The listing builds one solid part. Answer for the finished solid, in the listing's coordinates (mm). A direction names the side the tool comes from. Give positions to 0.01 mm unless a question says otherwise; leave off trailing zeros. Order: outer loops, then holes, each group sorted by start corner. A loop starts at its lowest first (then second) coordinate and runs counter-clockwise, first axis right, second up. Notation, with made-up numbers: (0.5, 21) - (13.5, 21) arc R26 cw to (13.5, 57) - close; hole circle Ø11 at (-36, 22). An arc over 180 degrees is marked (long way). Answer in a Markdown table with one row per item. Add a question column.
```python
from build123d import *

# Parameters (mm, degrees)
SKETCH1_W           = 68
SKETCH1_H           = 39.37
SKETCH1_R           = 4.25
BOSS_EXTRUDE1_DEPTH = 5
SKETCH2_W           = 68
SKETCH2_H           = 4.7625
BOSS_EXTRUDE2_DEPTH = 68
SKETCH4_R           = 3.15
CUT_EXTRUDE2_DEPTH  = 88.650893072
SKETCH14_R          = 23.5
CUT_EXTRUDE3_DEPTH  = 90.638144224


with BuildPart() as part:
    # Sketch1 → Boss-Extrude1 (new body)
    with BuildSketch(Plane(origin=(0, 0, 0), x_dir=(0, 0, -1), z_dir=(0, 1, 0))):
        Rectangle(SKETCH1_W, SKETCH1_H)
        with Locations(Location((-25, -2.735, 0), (0, 0, 180))):
            Circle(SKETCH1_R, mode=Mode.SUBTRACT)
        with Locations(Location((25, -2.735, 0), (0, 0, 180))):
            Circle(SKETCH1_R, mode=Mode.SUBTRACT)
    extrude(amount=BOSS_EXTRUDE1_DEPTH)

    # Sketch2 → Boss-Extrude2 (add)
    with BuildSketch(Plane(origin=(0, 5, 0), x_dir=(0, 0, -1), z_dir=(0, 1, 0))):
        with Locations((0, 17.30375)):
            Rectangle(SKETCH2_W, SKETCH2_H)
    extrude(amount=BOSS_EXTRUDE2_DEPTH)

    # Sketch4 → Cut-Extrude2 (cut, through all)
    with BuildSketch(Plane(origin=(-14.9225, 0, 0), x_dir=(0, 0, -1), z_dir=(1, 0, 0))):
        with Locations(Location((-27.577164466, 61.577164466, 0), (0, 0, 90))):
            Circle(SKETCH4_R)
        with Locations(Location((27.577164466, 61.577164466, 0), (0, 0, 90))):
            Circle(SKETCH4_R)
    extrude(amount=-CUT_EXTRUDE2_DEPTH, mode=Mode.SUBTRACT)

    # Sketch14 → Cut-Extrude3 (cut, through all)
    with BuildSketch(Plane.ZY.offset(19.685)):
        with Locations((0, 34)):
            Circle(SKETCH14_R)
    extrude(amount=-CUT_EXTRUDE3_DEPTH, mode=Mode.SUBTRACT)


solid = part.part
```
(1) Each of these flat-tipped pins is pushed along its axis until it touches: P1, Ø8, axis at x = 11, z = 26.5, coming from the +Y side; P2, Ø5, axis at y = 59, z = -27, coming from the +X side; P3, Ø5.5, axis at y = 61.58, z = 27.58, coming from the -X side. Where does it stop, or does it pass through?
(2) Find section C-C, the plane y = 34. Write down the section's boundary in (x, z) (1 decimal), plus the area to 3 significant figures.
(3) The mould has two halves that part along Y. Classify faces 1 (the face through (-17.34, 57.3, -3.06)), 2 (the face through (-1.414, 2.465, 24.079)), 3 (the face through (2, 5, 0)): +Y half, -Y half, draft (parallel to the pull), parting line (faces both ways), or undercut.
(4) Find section A-A, the plane y = 61.5. Write down the section's boundary in (x, z) (1 decimal).
(5) Find section D-D, the plane z = -19.5. Write down the section's boundary in (x, y) (1 decimal).
(6) Straight lines are drawn through the part: line 1 (Y direction, x = -15, z = 0); line 2 (Y direction, x = -0.5, z = -11.5); line 3 (X direction, y = 8, z = 23) (1 decimal). For each, find the intervals that lie inside material, in ascending order.
(7) For faces 4 (the face through (19.685, 2, 0)), 5 (the face through (-14.923, 54, 16)), determine the directions among +Z, -Z, +X, -X, +Y, -Y from which every point of the face is accessible in a straight line to the end or side of a thin tool.
(8) Find section B-B, the plane z = 0. Write down the section's boundary in (x, y) (1 decimal).
Answer key:
| question | item | result |
|---|---|---|
| 1 | P1 | y = 5 |
| 1 | P2 | x = -14.92 |
| 1 | P3 | through |
| 2 | outline | (-19.7, -34) - (-14.9, -34) - (-14.9, -23.5) - (-19.7, -23.5) - close; (-19.7, 23.5) - (-14.9, 23.5) - (-14.9, 34) - (-19.7, 34) - close |
| 2 | area | 100 mm² |
| 3 | face 1 | undercut |
| 3 | face 2 | draft |
| 3 | face 3 | +Y half |
| 4 | outline | (-19.7, -34) - (-14.9, -34) - (-14.9, -30.7) - (-19.7, -30.7) - close; (-19.7, -24.4) - (-14.9, -24.4) - (-14.9, 24.4) - (-19.7, 24.4) - close; (-19.7, 30.7) - (-14.9, 30.7) - (-14.9, 34) - (-19.7, 34) - close |
| 5 | outline | (-19.7, 0) - (19.7, 0) - (19.7, 5) - (-14.9, 5) - (-14.9, 20.9) - (-19.7, 20.9) - close; (-19.7, 47.1) - (-14.9, 47.1) - (-14.9, 73) - (-19.7, 73) - close |
| 6 | line 1 | 0 to 10.5, 57.5 to 73 |
| 6 | line 2 | 0 to 5 |
| 6 | line 3 | -19.7 to -14.9 |
| 7 | face 4 | +Z, -Z, +X, +Y, -Y |
| 7 | face 5 | +Z, -Z, +X, +Y |
| 8 | outline | (-19.7, 0) - (19.7, 0) - (19.7, 5) - (-14.9, 5) - (-14.9, 10.5) - (-19.7, 10.5) - close; (-19.7, 57.5) - (-14.9, 57.5) - (-14.9, 73) - (-19.7, 73) - close |
